from build123d import *

# Parameters (mm, degrees)
SKETCH2_W           = 90
SKETCH2_H           = 170
BOSS_EXTRUDE1_DEPTH = 10
SKETCH3_R           = 2.5
BOSS_EXTRUDE4_DEPTH = 6
SKETCH9_R           = 2.5
BOSS_EXTRUDE6_DEPTH = 15
SKETCH10_R          = 5
CUT_EXTRUDE3_DEPTH  = 15
FILLET1_R           = 10
FILLET2_R           = 10
FILLET3_R           = 10
FILLET4_R           = 10


with BuildPart() as part:
    # Sketch2 → Boss-Extrude1 (new body)
    with BuildSketch(Plane.XY):
        with Locations((45, 85)):
            Rectangle(SKETCH2_W, SKETCH2_H)
    extrude(amount=BOSS_EXTRUDE1_DEPTH)

    # Sketch3 → Boss-Extrude4 (add)
    with BuildSketch(Plane.XY.offset(10)):
        with Locations(Location((5, 160, 0), (0, 0, 180))):
            Circle(SKETCH3_R)
        with Locations(Location((85, 160, 0), (0, 0, 180))):
            Circle(SKETCH3_R)
        with Locations(Location((85, 10, 0), (0, 0, 180))):
            Circle(SKETCH3_R)
        with Locations(Location((5, 10, 0), (0, 0, 180))):
            Circle(SKETCH3_R)
    extrude(amount=BOSS_EXTRUDE4_DEPTH)

    # Boss-Extrude5 cone 1 section (through the dimple's axis) → Boss-Extrude5 (revolve)
    with BuildSketch(Plane(origin=(5, 160, 16), x_dir=(0, 1, 0), z_dir=(1, 0, 0))):
        Polygon((0, 0), (2.5, 0), (0, 1.953214066), align=None)
    revolve(axis=Axis((5, 160, 16), (0, 0, 1)))

    # Boss-Extrude5 cone 2 section (through the dimple's axis) → Boss-Extrude5 cone 2 (revolve)
    with BuildSketch(Plane(origin=(85, 160, 16), x_dir=(0, 1, 0), z_dir=(1, 0, 0))):
        Polygon((0, 0), (2.5, 0), (0, 1.953214066), align=None)
    revolve(axis=Axis((85, 160, 16), (0, 0, 1)))

    # Boss-Extrude5 cone 3 section (through the dimple's axis) → Boss-Extrude5 cone 3 (revolve)
    with BuildSketch(Plane(origin=(85, 10, 16), x_dir=(0, 1, 0), z_dir=(1, 0, 0))):
        Polygon((0, 0), (2.5, 0), (0, 1.953214066), align=None)
    revolve(axis=Axis((85, 10, 16), (0, 0, 1)))

    # Boss-Extrude5 cone 4 section (through the dimple's axis) → Boss-Extrude5 cone 4 (revolve)
    with BuildSketch(Plane(origin=(5, 10, 16), x_dir=(0, 1, 0), z_dir=(1, 0, 0))):
        Polygon((0, 0), (2.5, 0), (0, 1.953214066), align=None)
    revolve(axis=Axis((5, 10, 16), (0, 0, 1)))

    # Sketch9 → Boss-Extrude6 (add)
    with BuildSketch(Plane(origin=(0, 0, 0), x_dir=(-1, 0, 0), z_dir=(0, 0, -1))):
        with Locations((-45, 150)):
            Circle(SKETCH9_R)
    extrude(amount=BOSS_EXTRUDE6_DEPTH)

    # Sketch10 → Cut-Extrude3 (cut)
    with BuildSketch(Plane(origin=(0, 0, 0), x_dir=(-1, 0, 0), z_dir=(0, 0, -1))):
        with Locations((-45, 84.5110045)):
            Circle(SKETCH10_R)
    extrude(amount=-CUT_EXTRUDE3_DEPTH, mode=Mode.SUBTRACT)

    # Fillet1
    fillet1_edges = [part.edges().sort_by_distance(p)[0] for p in [
        (90, 170, 5),
    ]]
    fillet(fillet1_edges, radius=FILLET1_R)

    # Fillet2
    fillet2_edges = [part.edges().sort_by_distance(p)[0] for p in [
        (0, 170, 5),
    ]]
    fillet(fillet2_edges, radius=FILLET2_R)

    # Fillet3
    fillet3_edges = [part.edges().sort_by_distance(p)[0] for p in [
        (0, 0, 5),
    ]]
    fillet(fillet3_edges, radius=FILLET3_R)

    # Fillet4
    fillet4_edges = [part.edges().sort_by_distance(p)[0] for p in [
        (90, 0, 5),
    ]]
    fillet(fillet4_edges, radius=FILLET4_R)


solid = part.part
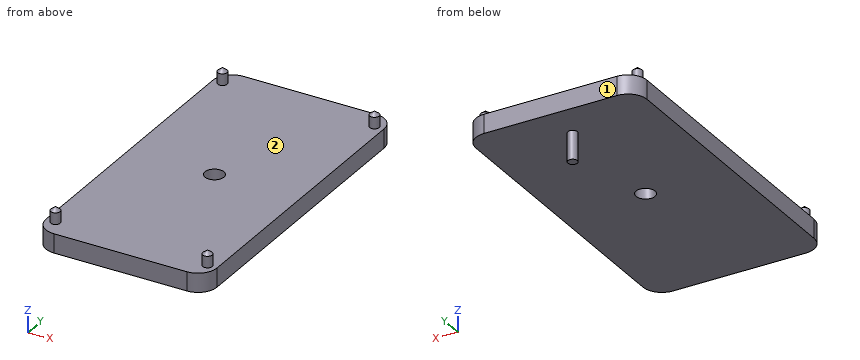
Can you work these out from the model? Positions are in its coordinate system, mm. Face numbers are marked on the shaded views. A direction names the side the tool comes from. Give positions to 0.01 mm unless a question says otherwise; leave off trailing zeros. Loops run counter-clockwise (first coordinate to the right, second up) from the corner with the lowest first, then second, coordinate; pieces in that order, holes last. Notation, with made-up numbers: M 14,8.25 L 43,8.25 A28 cw 43,34.25 Z; hole C 82,84 d5. An arc over 180 degrees is marked long. One line per item, written item: value. Start each with the question number.
1) On a 3-axis mill with a long thin cutter (end or side, diameter ignored), from which of +Z, -Z, +X, -X, +Y, -Y can I reach the whole of each face in a straight line? I mean the marked faces 1 and 2. Say none if no direction works.
2) I'm going to push flat-ended pins straight in: pin 1 (3 mm diameter, centred on x = 51.5, y = 77, fed in from +Z); pin 2 (2 mm diameter, centred on x = 80.5, y = 17, fed in from -Z). Where does each tip first touch, or does it pass through?
3) If I drill on line 1 (Y direction, x = 45, z = 4.25); line 2 (Z direction, x = 64.5, y = 45); line 3 (X direction, y = 82, z = 7.5), over which ranges is the centre line in solid material (lowest first)? Write a range as [from, to].
4) If we section it at B-B, the plane y = 150: Write out the boundary of the cut face in (x, z), and give its area (3 significant figures).
5) If we section it at C-C, the plane z = -4: Write out the boundary of the cut face in (x, y).
6) If we section it at A-A, the plane x = 45: Write out the boundary of the cut face in (y, z).
7) If we section it at D-D, the plane x = 31.5: Write out the boundary of the cut face in (y, z).
Completed:
1. face 1: +Z, -Z, +X, -X, +Y
1. face 2: +Z
2. pin 1: stops at z = 10
2. pin 2: stops at z = 0
3. line 1: y = [0, 79.51], [89.51, 170]
3. line 2: z = [0, 10]
3. line 3: x = [0, 40.68], [49.32, 90]
4. outline: M 0,0 L 42.5,0 L 42.5,-15 L 47.5,-15 L 47.5,0 L 90,0 L 90,10 L 0,10 Z
4. area: 975 mm^2
5. outline: C 45,150 d5
6. outline: M 0,0 L 79.51,0 L 79.51,10 L 0,10 Z; M 89.51,0 L 147.5,0 L 147.5,-15 L 152.5,-15 L 152.5,0 L 170,0 L 170,10 L 89.51,10 Z
7. outline: M 0,0 L 170,0 L 170,10 L 0,10 Z
